Geometry: final body of the model. Coordinates: model frame, mm. Face numbers are marked on the shaded views. A direction names the side the tool comes from. Round coordinates to 2 decimals unless told otherwise and drop trailing zeros. Loops run counter-clockwise (first coordinate to the right, second up) from the corner with the lowest first, then second, coordinate; pieces in that order, holes last. Notation, with made-up numbers: M 48,68.25 L 54,68.25 A11 ccw 54,76.25 Z; hole C -30,71.5 d11. An arc over 180 degrees is marked long. Answer as a JSON object with one key per item and string values.
```python
from build123d import *

# Parameters (mm, degrees)
SKETCH_1_R          = 42
EXTRUDE_1_DEPTH     = 3
SKETCH_2_W          = 11
SKETCH_2_H          = 11
EXTRUDE_2_DEPTH     = 4
SKETCH_4_R          = 6
CUT_EXTRUDE_1_DEPTH = 25
SKETCH_5_R          = 9
CUT_EXTRUDE_2_DEPTH = 9
CUT_EXTRUDE_START   = 8
SKETCH_6_R          = 10
SKETCH_6_R_2        = 9
CUT_EXTRUDE_3_DEPTH = 1.5
SKETCH_7_R          = 30
CUT_EXTRUDE_4_DEPTH = 30
FILLET_1_R          = 2
SKETCH_8_R          = 2.1
CUT_EXTRUDE_5_DEPTH = 120.624412224


with BuildPart() as part:
    # Sketch 1 → Extrude 1 (new body)
    with BuildSketch(Plane.XY):
        Circle(SKETCH_1_R)
    extrude(amount=EXTRUDE_1_DEPTH)



with BuildPart() as body_2:
    # Sketch 2 → Revolve 1 (revolve)
    with BuildSketch(Plane.XY.offset(3), mode=Mode.PRIVATE) as revolve_1_sk:
        with Locations((94.5, -0.125)):
            Rectangle(SKETCH_2_W, SKETCH_2_H)
    revolve(revolve_1_sk.sketch.rotate(Axis((100, 22.717290725, 3), (0, -1, 0)), 270), axis=Axis((100, 22.717290725, 3), (0, -1, 0)))


with BuildPart() as part_1:
    add(part.part)

    add(body_2.part)  # Extrude 2 merges body 2
    # Sketch 3 → Extrude 2 (add, symmetric)
    with BuildSketch(Plane.XY.offset(3)):
        with BuildLine():
            Line((17.314737244, 38.264864748), (90, 5.375))
            Line((90, 5.375), (90, -4))
            Line((90, -4), (17.911593748, -37.989140678))
            ThreePointArc((17.911593748, -37.989140678), (-41.998713488, -0.328732965), (17.314737244, 38.264864748))
        make_face()
    extrude(amount=EXTRUDE_2_DEPTH, both=True)

    # Sketch 4 → Cut-Extrude 1 (cut)
    with BuildSketch(Plane.XZ.offset(5.625)):
        with Locations(Location((100, 3, 0), (0, 0, 270))):
            Circle(SKETCH_4_R)
    extrude(amount=-CUT_EXTRUDE_1_DEPTH, mode=Mode.SUBTRACT)

    # Sketch 5 → Cut-Extrude 2 (cut)
    with BuildSketch(Plane.XZ.offset(5.625)):
        with Locations(Location((100, 3, 0), (0, 0, 270))):
            Circle(SKETCH_5_R)
    extrude(amount=-CUT_EXTRUDE_2_DEPTH, mode=Mode.SUBTRACT)

    # Sketch 6 → Cut-Extrude 3 (cut)
    # profile 1 of 2: a face of its own
    with BuildSketch(Plane.XZ.offset(-3.375).offset(CUT_EXTRUDE_START)):
        with Locations(Location((100, 3, 0), (0, 0, 270))):
            Circle(SKETCH_6_R)
        with Locations(Location((100, 3, 0), (0, 0, 270))):
            Circle(SKETCH_6_R_2, mode=Mode.SUBTRACT)
    # profile 2 of 2: a face of its own
    with BuildSketch(Plane.XZ.offset(-3.375).offset(CUT_EXTRUDE_START)):
        with Locations(Location((100, 3, 0), (0, 0, 270))):
            Circle(SKETCH_6_R_2)
    extrude(amount=-CUT_EXTRUDE_3_DEPTH, mode=Mode.SUBTRACT)

    # Sketch 7 → Cut-Extrude 4 (cut)
    with BuildSketch(Plane.XY.offset(7)):
        Circle(SKETCH_7_R)
        with BuildLine():
            Line((26.356552806, -27.373931471), (75.930900201, -4))
            Line((75.930900201, -4), (37.788887255, -4))
            ThreePointArc((37.788887255, -4), (34.135678377, -16.695971422), (26.356552806, -27.373931471))
        make_face()
        with BuildLine():
            Line((37.788887255, 4), (75.930900201, 4))
            Line((75.930900201, 4), (26.356552806, 27.373931471))
            ThreePointArc((26.356552806, 27.373931471), (34.135678377, 16.695971422), (37.788887255, 4))
        make_face()
    extrude(amount=-CUT_EXTRUDE_4_DEPTH, mode=Mode.SUBTRACT)

    # Fillet 1
    fillet_1_edges = [part_1.edges().sort_by_distance(p)[0] for p in [
        (37.788887255, 4, 3),
        (26.356552806, 27.373931471, 3),
        (75.930900201, 4, 3),
        (26.356552806, -27.373931471, 3),
        (37.788887255, -4, 3),
        (75.930900201, -4, 3),
    ]]
    fillet(fillet_1_edges, radius=FILLET_1_R)

    # Sketch 8 → Cut-Extrude 5 (cut, through all)
    with BuildSketch(Plane.XY.offset(7)):
        with Locations((14.110790662, 32.029448745)):
            Circle(SKETCH_8_R)
        with Locations((-3.794421191, 34.793711613)):
            Circle(SKETCH_8_R)
        with Locations((-20.682920951, 28.235027553)):
            Circle(SKETCH_8_R)
        with Locations((-32.029448745, 14.110790662)):
            Circle(SKETCH_8_R)
        with Locations((-34.793711613, -3.794421191)):
            Circle(SKETCH_8_R)
        with Locations((-28.235027553, -20.682920951)):
            Circle(SKETCH_8_R)
        with Locations((-14.110790662, -32.029448745)):
            Circle(SKETCH_8_R)
        with Locations((3.794421191, -34.793711613)):
            Circle(SKETCH_8_R)
        with Locations((20.682920951, -28.235027553)):
            Circle(SKETCH_8_R)
        with Locations((32.029448745, -14.110790662)):
            Circle(SKETCH_8_R)
        with Locations((34.793711613, 3.794421191)):
            Circle(SKETCH_8_R)
        with Locations((28.235027553, 20.682920951)):
            Circle(SKETCH_8_R)
    extrude(amount=-CUT_EXTRUDE_5_DEPTH, mode=Mode.SUBTRACT)


solid = part_1.part
```
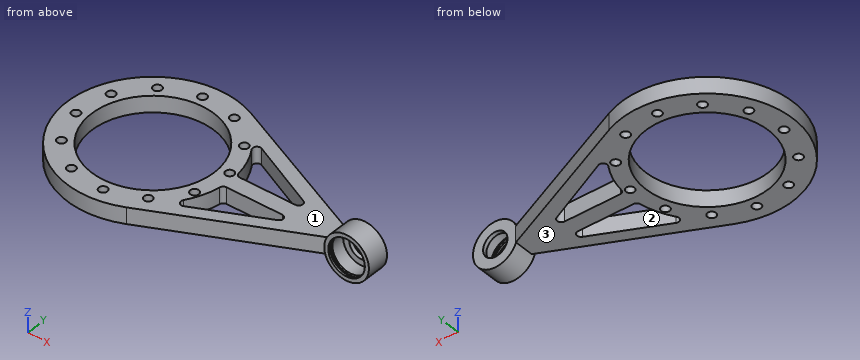
1) Cut plane A-A on y = 0. Return the cut outline in (x, z), and give its area (3 significant figures).
Geometry results:
{"outline": "M -42,-1 L -30,-1 L -30,7 L -42,7 Z; M 30,-1 L 89.75,-1 A11 ccw long 89.75,7 L 30,7 Z; hole C 100,3 d18", "area": "696 mm2"}
2) Cut plane B-B on x = 0. Return the cut outline in (y, z).
Geometry results:
{"outline": "M -42,-1 L -30,-1 L -30,7 L -42,7 Z; M 30,-1 L 42,-1 L 42,7 L 30,7 Z"}
3) Cut plane C-C on x = 100. Return the cut outline in (y, z) (3 decimals).
Geometry results:
{"outline": "M -5.625,-8 L 5.375,-8 L 5.375,-3 L 3.375,-3 L 3.375,-6 L -3.125,-6 L -3.125,-7 L -4.625,-7 L -4.625,-6 L -5.625,-6 Z; M -5.625,12 L -4.625,12 L -4.625,13 L -3.125,13 L -3.125,12 L 3.375,12 L 3.375,9 L 5.375,9 L 5.375,14 L -5.625,14 Z"}
4) Cut plane D-D on z = 0.75. Count the separate pieces of the cut face and the enclosed holes in it, and give its area (3 significant figures).
Geometry results:
{"separate pieces": "2", "enclosed holes": "15", "area": "3,600 mm2"}
5) First-contact query: pin 1 (10 mm diameter, centred on y = -16.5, z = 0, fed in from +X); pin 2 (5 mm diameter, centred on y = 11.5, z = -1.5, fed in from +X); pin 3 (10 mm diameter, centred on x = 105, z = -2, fed in from +Y) (3 decimals); pin 4 (4 mm diameter, centred on x = 32.03, y = -14.11, fed in from -Z). Flat tips, straight axial feed; report the tip coordinate or a pass-through.
Geometry results:
{"pin 1": "x = 74.09", "pin 2": "x = 81.88", "pin 3": "y = 5.375", "pin 4": "through"}
6) Set-up query: the marked faces 1, 2 and 3. Return all of +Z, -Z, +X, -X, +Y, -Y with unobstructed straight access to the full face (end or side cutting, diameter ignored); none if empty.
Geometry results:
{"face 1": "+Z, -X, +Y, -Y", "face 2": "+Z, -Z", "face 3": "-Z, -X, +Y, -Y"}
7) Line query: probe 1 along X at (y, z) = (1.25, 3); probe 2 along Y at (x, z) = (91, 1) (3 decimals); probe 3 along Y at (x, z) = (-19.5, 2). Output: solid intervals per line, ascending.
Geometry results:
{"probe 1": "-41.98 to -29.97, 29.97 to 91, 109 to 111", "probe 2": "-5.625 to -4.625, -3.125 to 5.375", "probe 3": "-37.2 to -22.8, 22.8 to 26.5, 29.97 to 37.2"}
